CAD build for the part. Positions are in the model's coordinates, mm. Face numbers are marked on the shaded views. A direction names the side the tool comes from. Give positions to 0.01 mm unless a question says otherwise; leave off trailing zeros. Loops run counter-clockwise (first coordinate to the right, second up) from the corner with the lowest first, then second, coordinate; pieces in that order, holes last. Notation, with made-up numbers: (49, 81.5) -> (57, 81.5) arc R10 ccw to (57, 88.5) -> close; hole circle Ø10 at (84, -38). An arc over 180 degrees is marked (long way). Use one line per item in the form item = value.
```python
from build123d import *

# Parameters (mm, degrees)
F0_W           = 38.1
F0_H           = 12.7
F1_DEPTH       = 11.1125
F2_W           = 38.1
F2_H           = 22.225
F3_DEPTH       = 12.7
F5_D           = 11.1125
F5_DEPTH       = 12.7
F5_CBORE_D     = 22.225
F5_CBORE_DEPTH = 6.35
F6_R           = 3.175


with BuildPart() as f1:
    # F0 (on Top) → F1 (new body)
    with BuildSketch(Plane.XY):
        with BuildLine():
            ThreePointArc((-16.910493, 6.898722), (-28.021043, -16.829595), (-16.373765, -40.299113))
            ThreePointArc((-16.373765, -40.299113), (2.139507, -46.649113), (20.652779, -40.299113))
            ThreePointArc((20.652779, -40.299113), (31.485209, -23.458425), (29.384606, -3.545168))
            Line((29.384606, -3.545168), (14.72239, -18.207384))
            ThreePointArc((14.72239, -18.207384), (-9.987481, -20.25837), (11.526728, -7.932662))
            Line((11.526728, -7.932662), (23.880181, 4.42079))
            Line((23.880181, 4.42079), (21.189507, 21.613387))
            Line((21.189507, 21.613387), (-16.910493, 21.613387))
            Line((-16.910493, 21.613387), (-16.910493, 6.898722))
        make_face()
        with Locations((2.139507, 27.963387)):
            Rectangle(F0_W, F0_H)
        with BuildLine():
            Line((-16.373765, -40.299113), (-32.785493, -40.299113))
            Line((-32.785493, -40.299113), (-32.785493, -48.236613))
            Line((-32.785493, -48.236613), (37.064507, -48.236613))
            Line((37.064507, -48.236613), (37.064507, -40.299113))
            Line((37.064507, -40.299113), (20.652779, -40.299113))
            ThreePointArc((20.652779, -40.299113), (2.139507, -46.649113), (-16.373765, -40.299113))
        make_face()
    extrude(amount=F1_DEPTH)

    # F2 (on face) → F3 (join)
    with BuildSketch(Plane(origin=(0, 34.313387, 0), x_dir=(-1, 0, 0), z_dir=(0, 1, 0))):
        with BuildLine():
            ThreePointArc((16.910493, 33.3375), (-2.139507, 52.3875), (-21.189507, 33.3375))
            Line((-21.189507, 33.3375), (16.910493, 33.3375))
        make_face()
        with Locations((-2.139507, 22.225)):
            Rectangle(F2_W, F2_H)
    extrude(amount=-F3_DEPTH)

    # F5
    with Locations(Plane.XZ.offset(-21.613387)):
        with Locations((2.139507, 33.3375)):
            CounterBoreHole(F5_D / 2, F5_CBORE_D / 2, F5_CBORE_DEPTH, depth=F5_DEPTH)

    # F6
    f6_edges = [f1.edges().sort_by_distance(p)[0] for p in [
        (37.064507, -40.299113, 5.55625),
        (20.652779, -40.299113, 5.55625),
        (-16.373765, -40.299113, 5.55625),
        (-32.785493, -40.299113, 5.55625),
    ]]
    fillet(f6_edges, radius=F6_R)


solid = f1.part
```
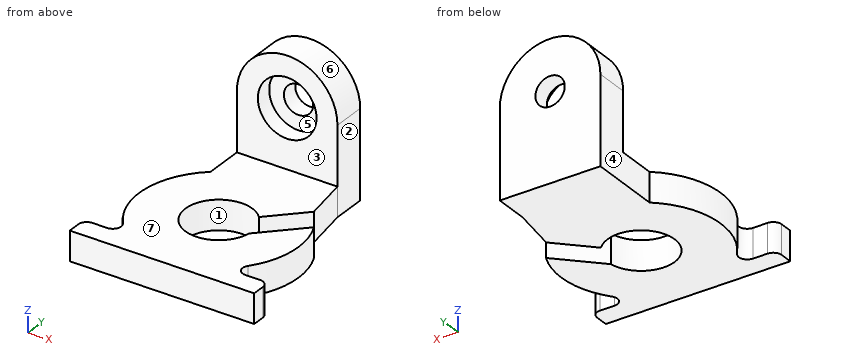
1. Drill centre lines: line 1 (Y direction, x = -10.5, z = 32.5); line 2 (Z direction, x = -10, y = -30.5); line 3 (X direction, y = -19, z = 3.5). Where is each one in solid material? Low to high.
Result sheet:
line_1 = 21.61 to 34.31
line_2 = 0 to 11.11
line_3 = -27.92 to -10.31, 14.59 to 32.2
2. Cut at B-B, the plane x = -6. Write the cut outline in (y, z), then the cut area to 3 significant figures.
Result sheet:
outline = (-48.24, 0) -> (-26.24, 0) -> (-26.24, 11.11) -> (-48.24, 11.11) -> close; (-6.74, 0) -> (34.31, 0) -> (34.31, 50.56) -> (21.61, 50.56) -> (21.61, 40.9) -> (27.96, 40.9) -> (27.96, 25.77) -> (21.61, 25.77) -> (21.61, 11.11) -> (-6.74, 11.11) -> close
area = 1,110 mm^2
3. Drop flat-ended pins along their axis: P1, Ø18, axis at x = 0, z = 35.5, coming from the -Y side; P2, Ø8, axis at y = 26, z = 8.5, coming from the -X side; P3, Ø18, axis at x = 2.14, z = 33.34, coming from the -Y side; P4, Ø1, axis at x = 12, y = -10, coming from the -Z side. Give the stop position or say it passes through.
Result sheet:
P1 = 21.61
P2 = -16.91
P3 = 27.96
P4 = through
4. Mould opens along Y. For the marked faces 1, 2 and 3 say: pulls with the +Y half, pulls with the -Y half, needs draft (parallel to the pull), parting line crosses it, or undercut.
Result sheet:
face_1 = undercut
face_2 = needs draft
face_3 = pulls with the -Y half
5. Cut at C-C, the plane z = 35. Write the cut outline in (x, y).
Result sheet:
outline = (-16.84, 21.61) -> (-8.85, 21.61) -> (-8.85, 27.96) -> (-3.16, 27.96) -> (-3.16, 34.31) -> (-16.84, 34.31) -> close; (7.44, 27.96) -> (13.13, 27.96) -> (13.13, 21.61) -> (21.12, 21.61) -> (21.12, 34.31) -> (7.44, 34.31) -> close
6. Tool access for the marked faces 4, 5, 6 and 7: list every direction of +Z, -Z, +X, -X, +Y, -Y with a clear straight run to the whole face (end or side of a thin tool).
Result sheet:
face_4 = +Z, -Z, -X, +Y
face_5 = -Y
face_6 = +Z, +Y, -Y
face_7 = +Z, +X, -X, -Y
7. Cut at A-A, the plane y = -11. Write the cut outline in (x, z), then the cut area to 3 significant figures.
Result sheet:
outline = (-27.52, 0) -> (-9.31, 0) -> (-9.31, 11.11) -> (-27.52, 11.11) -> close; (21.93, 0) -> (31.8, 0) -> (31.8, 11.11) -> (21.93, 11.11) -> close
area = 312 mm^2
